Part model, mm, in its own coordinate system. A direction names the side the tool comes from. Coordinates: 2 decimals unless noted, no trailing zeros. Write each loop counter-clockwise with the first axis right and the second up, starting at its lowest first coordinate (ties: lowest second). Pieces come first, ordered by that corner, then holes. Notation, with made-up numbers: (-3.75, -2) -> (53.25, -2) arc R23 cw to (53.25, 21) -> close; hole circle Ø4 at (9.5, 52.5). An arc over 180 degrees is marked (long way). One line per question, with ' | ' between items. Start each with the question number.
Item 1: Pin check, flat tips, straight feed: pin 1 (4 mm diameter, centred on x = 64, y = -17.5, fed in from -Z); pin 2 (1 mm diameter, centred on x = 75, z = 32.5, fed in from -Y); pin 3 (3 mm diameter, centred on x = 71, z = 1.5, fed in from -Y); pin 4 (2 mm diameter, centred on y = -35.5, z = -15, fed in from -X). Stop position of each tip, or through.
Item 2: Two-plate mould, pull along X, no slides. Class faces 1 (the cylindrical face through (57.52, -17.56, -42.35)), 2 (the conical face through (77.43, -4.32, -19.46)), 3 (the cylindrical face through (35.28, -9.04, 40.73)): pulls with the +X half, pulls with the -X half, needs draft (parallel to the pull), parting line crosses it, or undercut.
Item 3: 3-axis set-ups, long thin cutter, end or side, ignore diameter. For faces 4 (the cylindrical face through (15.65, -17.56, -42.35)), 5 (the cylindrical face through (80.21, -9.04, 40.73)): which of +Z, -Z, +X, -X, +Y, -Y reach the whole face in a straight line?
Item 4: Saw through at B-B (x = 68). List the corners of the cut face in (y, z).
Item 5: Saw through at A-A (x = 95.5). List the corners of the cut face in (y, z), and give its area (3 significant figures).
Item 6: Probe probe 1 along Z at (x, y) = (75, 16.5); probe 2 along Z at (x, y) = (91, -25); probe 3 along Y at (x, z) = (102, -29.5). List the from-to ranges inside material, lowest first. Write a range as [from, to].
from build123d import *

# Parameters (mm, degrees)
SKETCH1_R           = 45.847
BOSS_EXTRUDE1_DEPTH = 109.22


with BuildPart() as part:
    # Sketch1 → Boss-Extrude1 (new body)
    with BuildSketch(Plane(origin=(0, 0, 0), x_dir=(0, 0, -1), z_dir=(1, 0, 0))):
        Circle(SKETCH1_R)
    extrude(amount=BOSS_EXTRUDE1_DEPTH)

    # Sketch3 → Cut-Revolve1 (revolve, cut)
    with BuildSketch(Plane.XY):
        Polygon((0, 0), (0, 28.321), (58.298365665, 12.7), (64.77, 12.7), (109.22, 38.1), (109.22, 0), align=None)
    revolve(axis=Axis((0, 0, 0), (1, 0, 0)), mode=Mode.SUBTRACT)

    # Sketch4 → Cut-Revolve2 (revolve, cut)
    with BuildSketch(Plane.XY):
        with BuildLine():
            Line((76.6826, 45.847), (83.82, 45.847))
            Line((83.82, 45.847), (83.82, 42.4815))
            ThreePointArc((83.82, 42.4815), (83.596815367, 41.942684633), (83.058, 41.7195))
            Line((83.058, 41.7195), (77.4446, 41.7195))
            ThreePointArc((77.4446, 41.7195), (76.905784633, 41.942684633), (76.6826, 42.4815))
            Line((76.6826, 42.4815), (76.6826, 45.847))
        make_face()
        with BuildLine():
            Line((31.75, 45.847), (38.8874, 45.847))
            Line((38.8874, 45.847), (38.8874, 42.4815))
            ThreePointArc((38.8874, 42.4815), (38.664215367, 41.942684633), (38.1254, 41.7195))
            Line((38.1254, 41.7195), (32.512, 41.7195))
            ThreePointArc((32.512, 41.7195), (31.973184633, 41.942684633), (31.75, 42.4815))
            Line((31.75, 42.4815), (31.75, 45.847))
        make_face()
    revolve(axis=Axis((0, 0, 0), (-1, 0, 0)), mode=Mode.SUBTRACT)


solid = part.part
From the geometry:
1) pin 1: z = -43.15 | pin 2: y = -32.83 | pin 3: y = -45.85 | pin 4: x = 0
2) face 1: needs draft | face 2: pulls with the +X half | face 3: undercut
3) face 4: +X, -X | face 5: none
4) outline: circle Ø91.69 at (0, 0); hole circle Ø29.09 at (0, 0)
5) outline: circle Ø91.69 at (0, 0); hole circle Ø60.52 at (0, 0) | area: 3,730 mm2
6) probe 1: [-42.77, -8.47], [8.47, 42.77] | probe 2: [-38.43, -11.9], [11.9, 38.43] | probe 3: [-35.1, -16.85], [16.85, 35.1]
